```python
from build123d import *

# Parameters (mm, degrees)
F0_W      = 20
F0_H      = 40
F1_DEPTH  = 12
F2_R      = 3
F3_DEPTH  = 12
F5_DEPTH  = 23
F7_DEPTH  = 20
F8_R      = 1.99999
F9_R      = 1
F10_W     = 5.5
F10_H     = 10
F11_DEPTH = 25
F13_DEPTH = 1
F14_SIZE  = 0.5


# Not quite as in the source:
# - a fillet or chamfer is up to 0.001 mm smaller than in the source, because OpenCascade refuses the exact size


with BuildPart() as f1:
    # F0 (on Front) → F1 (new body)
    with BuildSketch(Plane.XZ):
        with Locations((10, 20)):
            Rectangle(F0_W, F0_H)
    extrude(amount=F1_DEPTH)

    # F2 (on face) → F3 (cut, through all)
    with BuildSketch(Plane(origin=(0, 0, 0), x_dir=(-1, 0, 0), z_dir=(0, 1, 0))):
        with Locations((-10, 30)):
            Circle(F2_R)
        with Locations((-10, 10)):
            Circle(F2_R)
    extrude(amount=-F3_DEPTH, mode=Mode.SUBTRACT)

    # F4 (on face) → F5 (join)
    with BuildSketch(Plane.XZ.offset(12)):
        Polygon((0, 4.2264973081), (0, 0), (20, 0), (20, 4.2264973081), (10, 10), align=None)
    extrude(amount=F5_DEPTH)

    # F6 (on face) → F7 (join, through all)
    with BuildSketch(Plane.YZ.offset(20)):
        Polygon((-35, 40), (-35, 4.2264973081), (-30, 4.2264973081), (-30, 35), (-12, 35), (-12, 40), align=None)
    extrude(amount=-F7_DEPTH)

    # F8 (radius 2 in the source; OpenCascade refuses exactly that, so slightly less here)
    f8_edges = [f1.edges().sort_by_distance(p)[0] for p in [
        (10, -35, 40),
        (10, -35, 0),
        (10, -30, 35),
        (10, -12, 35),
    ]]
    fillet(f8_edges, radius=F8_R)

    # F9
    f9_edges = [f1.edges().sort_by_distance(p)[0] for p in [
        (20, -35, 20),
        (0, -35, 20),
    ]]
    fillet(f9_edges, radius=F9_R)

    # F10 (on face) → F11 (cut)
    with BuildSketch(Plane.YZ.offset(20)):
        with Locations((-6.25, 30)):
            Rectangle(F10_W, F10_H)
        with Locations((-6.25, 10)):
            Rectangle(F10_W, F10_H)
    extrude(amount=-F11_DEPTH, mode=Mode.SUBTRACT)

    # F12 (on face) → F13 (cut)
    with BuildSketch(Plane.XZ.offset(35)):
        Polygon((16.5859262925, 23.9497199655), (3.0391060282, 23.9497199655), (3.0391060282, 21.5699486434), (9.6455384046, 21.5699486434), (9.8125161603, 21.5699486434), (16.5859262925, 21.5699486434), align=None)
        Polygon((9.8125161603, 21.5699486434), (9.6455384046, 21.5699486434), (7.6536308043, 16.2067040801), (12.2681558132, 16.2067040801), align=None)
    extrude(amount=-F13_DEPTH, mode=Mode.SUBTRACT)

    # F14
    f14_edges = [f1.edges().sort_by_distance(p)[0] for p in [
        (20, -12, 18.613254),
        (0, -12, 18.613254),
    ]]
    chamfer(f14_edges, length=F14_SIZE)


solid = f1.part
```
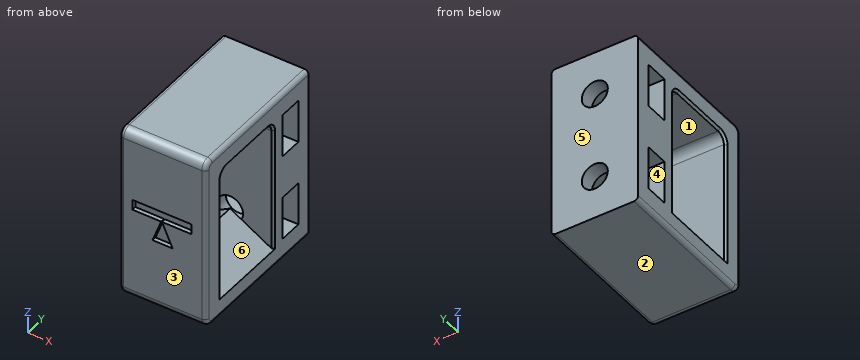
Work out the finished part from the listing and answer in its coordinate system (mm). Face numbers are marked on the shaded views. A direction names the side the tool comes from. Round coordinates to 2 decimals unless told otherwise and drop trailing zeros. Write each loop counter-clockwise with the first axis right and the second up, starting at its lowest first coordinate (ties: lowest second). Pieces come first, ordered by that corner, then holes.
1) Flat-ended cylindrical pins translate along their axes: P1, Ø1.5, axis at x = 10.5, z = 8, coming from the +Y side; P2, Ø0.5, axis at x = 13, y = -34.5, coming from the +Z side; P3, Ø0.5, axis at y = -34.5, z = 23.5, coming from the +X side. Find the tip coordinate at first contact, or state that the pin passes through.
2) A cutting plane is placed at C-C on y = -10.5. Determine the outline of the cut face in (x, z), and give its area (3 significant figures).
3) A cutting plane is placed at D-D on x = 5.75. Determine the outline of the cut face in (y, z), and give its area (3 significant figures).
4) Which of the six approach directions +Z, -Z, +X, -X, +Y, -Y give full straight-line access (tool end or side, diameter ignored) to the marked faces 4, 5 and 6?
5) Determine the mould class of the marked faces 1, 2 and 3 for opening direction Z: pulls with the +Z half, pulls with the -Z half, needs draft (parallel to the pull), parting line crosses it, or undercut.
6) A cutting plane is placed at B-B on y = -16. Determine the outline of the cut face in (x, z).
7) A cutting plane is placed at A-A on z = 30. Determine the outline of the cut face in (x, y), and give its area (3 significant figures).
8) Consider probe 1 along Z at (x, y) = (10, -10); probe 2 along Y at (x, z) = (19, 30.5); probe 3 along Y at (x, z) = (14, 6). Determine where each line is inside the solid, lowest interval first.
Entries:
1. P1: stops at y = -12
1. P2: stops at z = 39.56
1. P3: stops at x = 19.97
2. outline: (0, 1) arc R1 ccw to (1, 0) - (19, 0) arc R1 ccw to (20, 1) - (20, 39) arc R1 ccw to (19, 40) - (1, 40) arc R1 ccw to (0, 39) - close; hole circle Ø6 at (10, 10); hole circle Ø6 at (10, 30)
2. area: 743 mm2
3. outline: (-35, 2) arc R2 ccw to (-33, 0) - (0, 0) - (0, 40) - (-33, 40) arc R2 ccw to (-35, 38) - (-35, 23.95) - (-34, 23.95) - (-34, 21.57) - (-35, 21.57) - close; hole (-30, 7.55) - (-12, 7.55) - (-12, 33) arc R2 ccw to (-14, 35) - (-28, 35) arc R2 ccw to (-30, 33) - close; hole (-9, 5) - (-3.5, 5) - (-3.5, 15) - (-9, 15) - close; hole (-9, 25) - (-3.5, 25) - (-3.5, 35) - (-9, 35) - close
3. area: 793 mm2
4. face 4: +X, -X
4. face 5: +Z, -Z, +X, -X, +Y
4. face 6: +X
5. face 1: undercut
5. face 2: pulls with the -Z half
5. face 3: needs draft
6. outline: (0, 1) arc R1 ccw to (1, 0) - (19, 0) arc R1 ccw to (20, 1) - (20, 4.23) - (10, 10) - (0, 4.23) - close; (0, 35.5) - (0.5, 35) - (19.5, 35) - (20, 35.5) - (20, 39) arc R1 ccw to (19, 40) - (1, 40) arc R1 ccw to (0, 39) - close
7. outline: (0, -34) arc R1 ccw to (1, -35) - (19, -35) arc R1 ccw to (20, -34) - (20, -30.5) - (19.5, -30) - (0.5, -30) - (0, -30.5) - close; (0, -11.5) - (0.5, -12) - (7, -12) - (7, -9) - (0, -9) - close; (0, -3.5) - (7, -3.5) - (7, 0) - (0, 0) - close; (13, -12) - (19.5, -12) - (20, -11.5) - (20, -9) - (13, -9) - close; (13, -3.5) - (20, -3.5) - (20, 0) - (13, 0) - close
7. area: 190 mm2
8. probe 1: z = 0 to 7, 13 to 27, 33 to 40
8. probe 2: y = -35 to -30, -12 to -9, -3.5 to 0
8. probe 3: y = -35 to -9, -3.5 to 0
